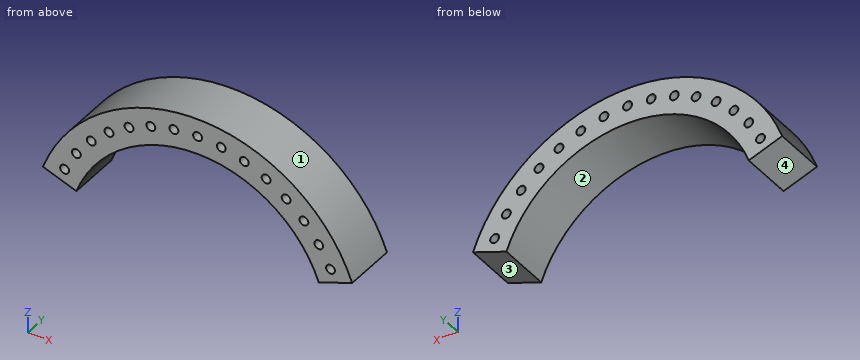
from build123d import *

# Parameters (mm, degrees)
BOSS_EXTRUDE1_DEPTH        = 38.1
F_1_4_0_2500_DOWEL_HOLE1_D = 6.35
CIRPATTERN1_COUNT          = 8
CIRPATTERN1_ANGLE          = 65
MIRROR1_COPY_1_D           = 6.35
MIRROR1_COPY_2_D           = 6.35
MIRROR1_COPY_3_D           = 6.35
MIRROR1_COPY_4_D           = 6.35
MIRROR1_COPY_5_D           = 6.35
MIRROR1_COPY_6_D           = 6.35
MIRROR1_COPY_7_D           = 6.35
MIRROR1_COPY_8_D           = 6.35


with BuildPart() as part:
    # Sketch1 → Boss-Extrude1 (new body)
    with BuildSketch(Plane(origin=(0, 0, 0), x_dir=(1, 0, 0), z_dir=(0, 1, 0))):
        with BuildLine():
            Line((-110.390390627, -40.178816337), (-86.522198059, -31.491504697))
            ThreePointArc((-86.522198059, -31.491504697), (0, -92.075), (86.522198059, -31.491504697))
            Line((86.522198059, -31.491504697), (110.390390627, -40.178816337))
            ThreePointArc((110.390390627, -40.178816337), (0, -117.475), (-110.390390627, -40.178816337))
        make_face()
    extrude(amount=-BOSS_EXTRUDE1_DEPTH)

    # 1/4 (0.2500) Dowel Hole1 (through all)
    with Locations(Plane(origin=(0, 0, 0), x_dir=(1, 0, 0), z_dir=(0, 1, 0))):
        with Locations((0, -104.775)):
            f_1_4_0_2500_dowel_hole1 = Hole(F_1_4_0_2500_DOWEL_HOLE1_D / 2)

    # CirPattern1: 1/4 (0.2500) Dowel Hole1 ×8 about axis
    cirpattern1_axis = Axis((0, 0, 0), (0, -1, 0))
    for i in range(1, CIRPATTERN1_COUNT):
        add(f_1_4_0_2500_dowel_hole1.rotate(cirpattern1_axis, i * CIRPATTERN1_ANGLE / (CIRPATTERN1_COUNT - 1)), mode=Mode.SUBTRACT)

    # Mirror1 copy 1 (through all)
    with Locations(Plane(origin=(0, 0, 0), x_dir=(-0.9868959788567211, 0, 0.161357760632807), z_dir=(0, 1, 0))):
        with Locations((0, 104.775)):
            Hole(MIRROR1_COPY_1_D / 2)

    # Mirror1 copy 2 (through all)
    with Locations(Plane(origin=(0, 0, 0), x_dir=(-0.9479273461671315, 0, 0.3184866502516851), z_dir=(0, 1, 0))):
        with Locations((0, 104.775)):
            Hole(MIRROR1_COPY_2_D / 2)

    # Mirror1 copy 3 (through all)
    with Locations(Plane(origin=(0, 0, 0), x_dir=(-0.8841153935046093, 0, 0.4672686282730629), z_dir=(0, 1, 0))):
        with Locations((0, 104.775)):
            Hole(MIRROR1_COPY_3_D / 2)

    # Mirror1 copy 4 (through all)
    with Locations(Plane(origin=(0, 0, 0), x_dir=(-0.7971325072229216, 0, 0.6038044103254785), z_dir=(0, 1, 0))):
        with Locations((0, 104.775)):
            Hole(MIRROR1_COPY_4_D / 2)

    # Mirror1 copy 5 (through all)
    with Locations(Plane(origin=(0, 0, 0), x_dir=(-0.6892583384839459, 0, 0.7245156608592739), z_dir=(0, 1, 0))):
        with Locations((0, 104.775)):
            Hole(MIRROR1_COPY_5_D / 2)

    # Mirror1 copy 6 (through all)
    with Locations(Plane(origin=(0, 0, 0), x_dir=(-0.5633200580636203, 0, 0.8262387743159961), z_dir=(0, 1, 0))):
        with Locations((0, 104.775)):
            Hole(MIRROR1_COPY_6_D / 2)

    # Mirror1 copy 7 (through all)
    with Locations(Plane(origin=(0, 0, 0), x_dir=(-0.4226182617406972, 0, 0.906307787036651), z_dir=(0, 1, 0))):
        with Locations((0, 104.775)):
            Hole(MIRROR1_COPY_7_D / 2)

    # Mirror1 copy 8 (through all)
    with Locations(Plane(origin=(0, 0, 0), x_dir=(-1, 0, 0), z_dir=(0, 1, 0))):
        with Locations((0, 104.775)):
            Hole(MIRROR1_COPY_8_D / 2)


solid = part.part
Source: CAD feature listing. Evaluate the final solid. Frame: model axes, mm. Face numbers are marked on the shaded views. Give positions to 0.01 mm unless a question says otherwise; leave off trailing zeros. Write each loop counter-clockwise with the first axis right and the second up, starting at its lowest first coordinate (ties: lowest second). Pieces come first, ordered by that corner, then holes. Notation, with made-up numbers: M 70.25,59 L 102.25,59 A36 cw 102.25,94 Z; hole C 23,16 d5. An arc over 180 degrees is marked long. Answer as a JSON object with one key per item and string values.
Q1. Cut plane B-B, the plane z = 52. Return the cut outline in (x, y).
Geometry check:
{"outline": "M -105.34,-38.1 L -75.99,-38.1 L -75.99,0 L -105.34,0 Z; M 75.99,-38.1 L 105.34,-38.1 L 105.34,0 L 75.99,0 Z"}
Q2. Cut plane A-A, the plane x = 0. Return the cut outline in (y, z) (3 decimals), then the cut area to 3 significant figures.
Geometry check:
{"outline": "M -38.1,92.075 L 0,92.075 L 0,101.6 L -38.1,101.6 Z; M -38.1,107.95 L 0,107.95 L 0,117.475 L -38.1,117.475 Z", "area": "726 mm^2"}
Q3. Ray query, line 1 along X through (y, z) = (-14, 47); line 2 along X through (y, z) = (-25.5, 94); line 3 along X through (y, z) = (-32.5, 83.5). Return the intervals inside material, ascending.
Geometry check:
{"line 1": "x = -107.66 to -96.6, -93.32 to -79.18, 79.18 to 93.32, 96.6 to 107.66", "line 2": "x = -70.46 to -51.82, -46.09 to 46.09, 51.82 to 70.46", "line 3": "x = -82.63 to -66.44, -60.09 to -38.8, 38.8 to 60.09, 66.44 to 82.63"}
Q4. Contact query for flat-ended pins moving along their axis: P1, Ø10, axis at y = -13, z = 94.5, coming from the -X side; P2, Ø12, axis at x = -56, y = -12, coming from the -Z side; P3, Ø6, axis at x = -67, y = -30, coming from the -Z side; P4, Ø5, axis at x = 48.96, z = 92.63, coming from the -Y side. Output: stop coordinate, or through.
Geometry check:
{"P1": "stops at x = -76.09", "P2": "stops at z = 68.07", "P3": "stops at z = 59.81", "P4": "passes through"}
Q5. Cut plane C-C, the plane y = -23. Count the separate pieces of the cut face and the enclosed holes in it, then the cut area to 3 significant figures.
Geometry check:
{"separate pieces": "1", "enclosed holes": "15", "area": "6,030 mm^2"}
Q6. Mould query, pull axis X, two halves, no side actions, for the marked faces 1, 2, 3 and 4. Classes: +X half, -X half, draft (parallel to the pull), parting line (faces both ways), or undercut.
Geometry check:
{"face 1": "parting line", "face 2": "undercut", "face 3": "+X half", "face 4": "-X half"}
